Design review of the part built by this model. Coordinates are the model's own, in mm. Face numbers are marked on the shaded views. A direction names the side the tool comes from. Coordinates: 2 decimals unless noted, no trailing zeros. Order: outer loops, then holes, each group sorted by start corner. A loop starts at its lowest first (then second) coordinate and runs counter-clockwise, first axis right, second up. Notation, with made-up numbers: (19, 59.5) -> (34, 59.5) arc R24 cw to (34, 86.5) -> close; hole circle Ø11 at (-0.5, 21.5). An arc over 180 degrees is marked (long way). Use a Markdown table: item, result. Add a question column.
Q1. Wall thickness on probe 1 along Z at (x, y) = (-0.25, 0); probe 2 along Z at (x, y) = (0.3, 0); probe 3 along Y at (x, z) = (0.3, 0): over which ranges is each line inside the solid? List them lowest first.
Q2. Add section B-B (y = -16). State the section outline as (x, z) points, then the cut area to 3 significant figures.
Q3. The part is to be moulded in two halves that separate along Y. For the marked faces 4 and 5, say which applies: pulls with the +Y half, pulls with the -Y half, needs draft (parallel to the pull), parting line crosses it, or undercut.
Q4. Add section C-C (x = -5.25). State the section outline as (y, z) points, then the cut area to 3 significant figures.
Q5. Add section D-D (y = -11). State the section outline as (x, z) points.
Q6. Add section A-A (z = -1.5). State the section outline as (x, y) points.
Q7. Machinability: for the marked faces 1, 2 and 3, which of the approach directions +Z, -Z, +X, -X, +Y, -Y give a long, thin tool a straight path to every point of the face, cutting with its end or side? Answer none if there is none.
Q8. Insertion check: pin 1 (3 mm diameter, centred on y = -5.5, z = 0, fed in from -X); pin 2 (0.6 mm diameter, centred on y = 5.5, z = 1.5, fed in from -X); pin 3 (10 mm diameter, centred on x = 1, y = -16.5, fed in from +Z); pin 4 (6 mm diameter, centred on x = -1, y = -1.5, fed in from -Z). Each pin has a flat end and moves straight along its axis. Give the tip position at first contact, or say it passes through.
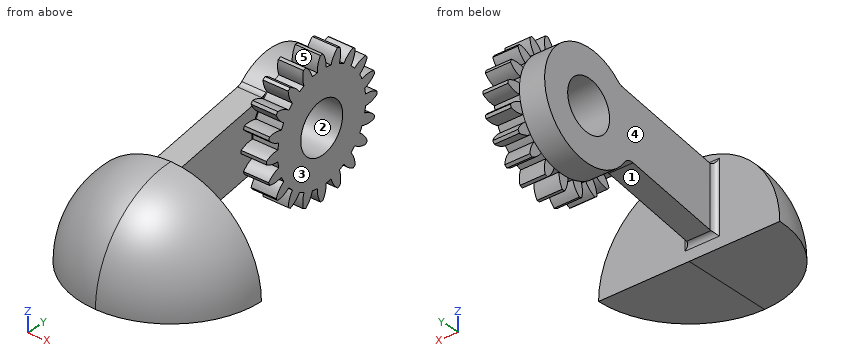
from build123d import *
from build123d.topology import SkipClean

# Parameters (mm, degrees)
BASPROSKE_W               = 2.5
BASPROSKE_H               = 6.6
TOOTHCUT_DEPTH            = 10.662815325
TEETHCUTS_COUNT           = 20
TEETHCUTS_ANGLE           = 342
HUBNEARONE_START          = 2.5000508
HUBNEAONESKE_R            = 5.249
HUBNEARONE_DEPTH          = 2.5000508
BORSKE_R                  = 2.5
BORE_DEPTH                = 5.0000508
MOVE_BODY_1_ANGLE         = 9
REVOLVE_1_ANGLE           = 90
REVOLVE_1_OTHER_WAY_ANGLE = 90
EXTRUDE_1_DEPTH           = 2.4
FILLET_1_R                = 1
FILLET_2_R                = 0.5


with BuildPart() as part:
    # BasProSke → Base-Revolve (revolve)
    with BuildSketch(Plane(origin=(0, 0, 0), x_dir=(1, 0, 0), z_dir=(0, 1, 0)), mode=Mode.PRIVATE) as base_revolve_sk:
        with Locations((1.25, 3.3)):
            Rectangle(BASPROSKE_W, BASPROSKE_H)
    revolve(base_revolve_sk.sketch.rotate(Axis((-10, 0, 0), (1, 0, 0)), 180), axis=Axis((-10, 0, 0), (1, 0, 0)))

    # TooCutSke → ToothCut (cut, through all)
    with BuildSketch(Plane(origin=(0, 0, 0), x_dir=(0, 0, -1), z_dir=(1, 0, 0))):
        with BuildLine():
            ThreePointArc((0.300213811, 5.240407681), (0, 5.249), (-0.300213811, 5.240407681))
            ThreePointArc((-0.300213811, 5.240407681), (-0.497369534, 5.948676387), (-0.899680168, 6.564030831))
            ThreePointArc((-0.899680168, 6.564030831), (0, 6.6254), (0.899680168, 6.564030831))
            ThreePointArc((0.899680168, 6.564030831), (0.497369534, 5.948676387), (0.300213811, 5.240407681))
        make_face()
    toothcut = extrude(amount=TOOTHCUT_DEPTH, mode=Mode.SUBTRACT)

    # TeethCuts: ToothCut ×20 about axis
    teethcuts_axis = Axis((-10, 0, 0), (1, 0, 0))
    for i in range(1, TEETHCUTS_COUNT):
        add(toothcut.rotate(teethcuts_axis, i * TEETHCUTS_ANGLE / (TEETHCUTS_COUNT - 1)), mode=Mode.SUBTRACT)

    # HubNeaOneSke → HubNearOne (add)
    with SkipClean():  # the faces are left unmerged after this step: merging them gives an invalid solid
        with BuildSketch(Plane.ZY.offset(HUBNEARONE_START)):
            Circle(HUBNEAONESKE_R)
        extrude(amount=-HUBNEARONE_DEPTH)

    # BorSke → Bore (cut, symmetric)
    with SkipClean():  # the faces are left unmerged after this step: merging them gives an invalid solid
        with BuildSketch(Plane(origin=(0, 0, 0), x_dir=(0, 0, -1), z_dir=(1, 0, 0))):
            with Locations(Location((0, 0, 0), (0, 0, 180))):
                Circle(BORSKE_R)
        extrude(amount=BORE_DEPTH, both=True, mode=Mode.SUBTRACT)


with BuildPart() as part_1:
    # Move Body 1: moved
    add(part.part.rotate(Axis((0, 0, 0), (-1, 0, 0)), MOVE_BODY_1_ANGLE))



with BuildPart() as body_2:
    # Sketch 4 → Revolve 1 (revolve)
    with BuildSketch(Plane(origin=(0, -5.800690391, 0.605708681), x_dir=(0, 0, -1), z_dir=(1, 0, 0))):
        with BuildLine():
            Line((6.405708681, -9.199309609), (6.405708681, -18.199309609))
            ThreePointArc((6.405708681, -18.199309609), (0.04174765, -15.56327064), (-2.594291319, -9.199309609))
            Line((-2.594291319, -9.199309609), (6.405708681, -9.199309609))
        make_face()
    revolve(axis=Axis((0, -15, -5.8), (0, -1, 0)), revolution_arc=REVOLVE_1_ANGLE)

    # Sketch 4 → Revolve 1 other way (revolve)
    with SkipClean():  # the faces are left unmerged after this step: merging them gives an invalid solid
        with BuildSketch(Plane(origin=(0, -5.800690391, 0.605708681), x_dir=(0, 0, -1), z_dir=(1, 0, 0))):
            with BuildLine():
                Line((6.405708681, -9.199309609), (6.405708681, -18.199309609))
                ThreePointArc((6.405708681, -18.199309609), (0.04174765, -15.56327064), (-2.594291319, -9.199309609))
                Line((-2.594291319, -9.199309609), (6.405708681, -9.199309609))
            make_face()
        revolve(axis=Axis((0, -15, -5.8), (0, 1, 0)), revolution_arc=REVOLVE_1_OTHER_WAY_ANGLE)


with BuildPart() as part_2:
    with SkipClean():  # the faces are left unmerged after this step: merging them gives an invalid solid
        add(part_1.part)

        add(body_2.part)  # Extrude 1 merges body 2
        # Sketch 5 → Extrude 1 (add)
        with BuildSketch(Plane.ZY.offset(2.5000508)):
            with BuildLine():
                Line((-4.3, -15), (-2.38467349, -4.137643583))
                ThreePointArc((-2.38467349, -4.137643583), (0.97980655, -4.674049764), (3.845615938, -2.83160734))
                Line((3.845615938, -2.83160734), (1.7, -15))
                Line((1.7, -15), (-4.3, -15))
            make_face()
        extrude(amount=-EXTRUDE_1_DEPTH)

    # Fillet 1
    fillet_1_edges = [part_2.edges().sort_by_distance(p)[0] for p in [
        (-1.3000508, -4.630675276, -2.471608279),
        (-1.3000508, -3.737073108, 3.685957893),
    ]]
    fillet(fillet_1_edges, radius=FILLET_1_R)

    # Fillet 2
    fillet_2_edges = [part_2.edges().sort_by_distance(p)[0] for p in [
        (-0.1000508, -15, -1.3),
        (-1.3000508, -15, 1.7),
        (-1.3000508, -15, -4.3),
        (-2.5000508, -15, -1.3),
    ]]
    fillet(fillet_2_edges, radius=FILLET_2_R)


solid = part_2.part
Established:
| question | item | result |
|---|---|---|
| 1 | probe 1 | -5.25 to -2.5, 2.5 to 5.25 |
| 1 | probe 2 | -6.6 to -2.5, 2.5 to 6.6 |
| 1 | probe 3 | -21.88 to -14.99, -6.6 to -2.5, 2.5 to 6.6 |
| 2 | outline | (-8.94, -5.8) -> (8.94, -5.8) arc R8.94 ccw to start |
| 2 | area | 126 mm^2 |
| 3 | face 4 | needs draft |
| 3 | face 5 | undercut |
| 4 | outline | (-22.31, -5.8) -> (-15, -5.8) -> (-15, 1.51) arc R7.31 ccw to start |
| 4 | area | 42.0 mm^2 |
| 5 | outline | (-2.5, -3.59) -> (-0.1, -3.59) -> (-0.1, 2.41) -> (-2.5, 2.41) -> close |
| 6 | outline | (-7.91, -15) arc R7.91 ccw to (7.91, -15) -> (0.4, -15) arc R0.5 cw to (-0.1, -14.5) -> (-0.1, -5.03) -> (0, -5.03) -> (0, -5.91) -> (2.5, -5.91) -> (2.5, -2) -> (-2.5, -2) -> (-2.5, -14.5) arc R0.5 cw to (-3, -15) -> close; (-2.5, 2) -> (2.5, 2) -> (2.5, 5.91) -> (0, 5.91) -> (0, 5.03) -> (-2.5, 5.03) -> close |
| 7 | face 1 | -Z, +X, -X |
| 7 | face 2 | +X, -X |
| 7 | face 3 | +Z, -Z, +X, +Y |
| 8 | pin 1 | x = -2.5 |
| 8 | pin 2 | x = 0 |
| 8 | pin 3 | z = 3.2 |
| 8 | pin 4 | z = -6.6 |
